For this review, take the finished solid that the model builds, in its own axes (mm). Coordinates: 2 decimals unless noted, no trailing zeros. Loops run counter-clockwise (first coordinate to the right, second up) from the corner with the lowest first, then second, coordinate; pieces in that order, holes last. Notation, with made-up numbers: (17.5, 7) - (24.5, 7) arc R21 cw to (24.5, 42) - close; hole circle Ø3 at (7, 88). An arc over 180 degrees is marked (long way). Use one line per item in the form item = value. Start each with the question number.
1. Add section C-C on z = 4. Give the boundary of the cut face in (x, y).
2. Add section A-A on z = -4. Give the boundary of the cut face in (x, y).
3. To check wall thickness, follow probe 1 along Z at (x, y) = (-32.5, -25.35); probe 2 along Y at (x, z) = (-32.4, -0.75); probe 3 along Y at (x, z) = (-32.15, -2.25). State the ranges of each line that lie inside material, in increasing order.
4. For pin 1 Ø0.5 at (y, z) = (-25, 3.5) entering from -X, flat-tipped, find the tip position at first contact; note if it passes through.
5. Add section B-B on y = -25. Give the boundary of the cut face in (x, z).
```python
from build123d import *

# Parameters (mm, degrees)
BOSS_EXTRUDE1_DEPTH      = 3
BOSS_EXTRUDE1_DEPTH_BACK = 10
SKETCH1_R                = 1
CHAMFER1_SIZE            = 0.5
CHAMFER1_SIZE2           = 1.743707222
BOSS_EXTRUDE2_DEPTH      = 0.1
BOSS_EXTRUDE2_DEPTH_BACK = 0.1


with BuildPart() as part:
    # Sketch1 → Boss-Extrude1 (new, two sides: drawn at the far end of the back side and taken through both)
    with BuildSketch(Plane.XY.offset(-BOSS_EXTRUDE1_DEPTH_BACK)):
        with Locations((-32.5, -25)):
            Circle(SKETCH1_R)
    extrude(amount=BOSS_EXTRUDE1_DEPTH + BOSS_EXTRUDE1_DEPTH_BACK)

    # Chamfer1
    chamfer1_edges = [part.edges().sort_by_distance(p)[0] for p in [
        (-33.5, -25, 3),
    ]]
    chamfer1_side = [part.faces().sort_by_distance(p)[0] for p in [
        (-32.5, -25, 3),
    ]]
    chamfer(chamfer1_edges, length=CHAMFER1_SIZE, length2=CHAMFER1_SIZE2, reference=chamfer1_side[0])

    # Sketch2 → Boss-Extrude2 (add, two sides: drawn at the far end of the back side and taken through both)
    with BuildSketch(Plane.ZY.offset(32.5).offset(-BOSS_EXTRUDE2_DEPTH_BACK)):
        Polygon((1.471640108, -25.31784203), (4.848999991, -25.31784203), (3.30552546, -24.648450588), (1.471640108, -24.648450588), align=None)
    extrude(amount=BOSS_EXTRUDE2_DEPTH + BOSS_EXTRUDE2_DEPTH_BACK)


solid = part.part
```
Conclusion:
q1.outline = (-32.6, -25.32) - (-32.4, -25.32) - (-32.4, -24.95) - (-32.6, -24.95) - close
q2.outline = circle Ø2 at (-32.5, -25)
q3.probe_1 = -10 to 3
q3.probe_2 = -25.99 to -24.01
q3.probe_3 = -25.94 to -24.06
q4.pin_1 = -32.6
q5.outline = (-33.5, -10) - (-31.5, -10) - (-31.5, 1.26) - (-32, 3) - (-32.4, 3) - (-32.4, 4.12) - (-32.6, 4.12) - (-32.6, 3) - (-33, 3) - (-33.5, 1.26) - close
